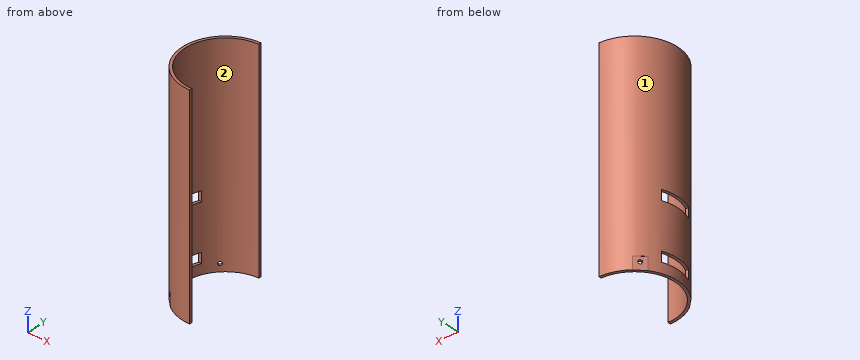
```python
from build123d import *

# Parameters (mm, degrees)
BOSS_EXTRUDE1_DEPTH      = 250
M4_CLEARANCE_HOLE1_D     = 4.5
M4_CLEARANCE_HOLE1_DEPTH = 15
M4_CLEARANCE_HOLE1_TIP   = 1.351936393
M4_CLEARANCE_HOLE2_D     = 4.5
M4_CLEARANCE_HOLE2_DEPTH = 15
M4_CLEARANCE_HOLE2_TIP   = 1.351936393
SKETCH9_W                = 12
SKETCH9_H                = 19.5
CUT_EXTRUDE1_DEPTH       = 10
CUT_EXTRUDE2_DEPTH       = 15
CIRPATTERN1_COUNT        = 2
CIRPATTERN1_ANGLE        = 270
CUT_EXTRUDE4_DEPTH       = 251.0000001


with BuildPart() as part:
    # Sketch1 → Boss-Extrude1 (new body)
    with BuildSketch(Plane.XY):
        with BuildLine():
            Line((0, 50.8), (0, 47.62))
            ThreePointArc((0, 47.62), (-47.62, 0), (0, -47.62))
            Line((0, -47.62), (0, -50.8))
            ThreePointArc((0, -50.8), (-50.8, 0), (0, 50.8))
        make_face()
    extrude(amount=BOSS_EXTRUDE1_DEPTH)

    # M4 Clearance Hole1
    with Locations(Plane(origin=(-35.921024484, 35.921024484, 0), x_dir=(0, 0, -1), z_dir=(-0.707106781, 0.707106781, 0))):
        with Locations((-9, 0)):
            Hole(M4_CLEARANCE_HOLE1_D / 2, depth=M4_CLEARANCE_HOLE1_DEPTH)
            with Locations((0, 0, -(M4_CLEARANCE_HOLE1_DEPTH + M4_CLEARANCE_HOLE1_TIP / 2))):  # 118° drill point
                Cone(0, M4_CLEARANCE_HOLE1_D / 2, M4_CLEARANCE_HOLE1_TIP, mode=Mode.SUBTRACT)

    # M4 Clearance Hole2
    with Locations(Plane(origin=(-35.921024484, -35.921024484, 0), x_dir=(0, 0, -1), z_dir=(-0.707106781, -0.707106781, 0))):
        with Locations((-9, 0)):
            Hole(M4_CLEARANCE_HOLE2_D / 2, depth=M4_CLEARANCE_HOLE2_DEPTH)
            with Locations((0, 0, -(M4_CLEARANCE_HOLE2_DEPTH + M4_CLEARANCE_HOLE2_TIP / 2))):  # 118° drill point
                Cone(0, M4_CLEARANCE_HOLE2_D / 2, M4_CLEARANCE_HOLE2_TIP, mode=Mode.SUBTRACT)

    # Sketch9 → Cut-Extrude1 (cut)
    with BuildSketch(Plane.ZY.offset(50.8)):
        with Locations((84, 9.75)):
            Rectangle(SKETCH9_W, SKETCH9_H)
        with Locations((84, -9.75)):
            Rectangle(SKETCH9_W, SKETCH9_H)
        Polygon((12, -19.5), (12, 0), (12, 19.5), (24, 19.5), (24, -19.5), align=None)
    extrude(amount=-CUT_EXTRUDE1_DEPTH, mode=Mode.SUBTRACT)

    # Sketch14 → Cut-Extrude2 (cut)
    with BuildSketch(Plane(origin=(0, 0, 0), x_dir=(-1, 0, 0), z_dir=(0, 0, -1))):
        with BuildLine():
            ThreePointArc((39.283322842, 32.206077218), (37.648654114, 34.102634894), (35.922518496, 35.916340685))
            Line((35.922518496, 35.916340685), (35.747788936, 35.741611124))
            Line((35.747788936, 35.741611124), (39.283322842, 32.206077218))
        make_face()
        with BuildLine():
            Line((35.747788936, 35.741611124), (35.922518496, 35.916340685))
            ThreePointArc((35.922518496, 35.916340685), (34.105872379, 37.645721305), (32.206077218, 39.283322842))
            Line((32.206077218, 39.283322842), (35.747788936, 35.741611124))
        make_face()
        with BuildLine():
            ThreePointArc((40.594896689, 30.540045233), (38.353880463, 33.310956958), (35.924113257, 35.917935446))
            Line((35.924113257, 35.917935446), (35.922518496, 35.916340685))
            ThreePointArc((35.922518496, 35.916340685), (37.648654114, 34.102634894), (39.283322842, 32.206077218))
            Line((39.283322842, 32.206077218), (35.747788936, 35.741611124))
            Line((35.747788936, 35.741611124), (35.570559867, 35.564382055))
            Line((35.570559867, 35.564382055), (40.594896689, 30.540045233))
        make_face()
        with BuildLine():
            Line((35.922518496, 35.916340685), (35.924113257, 35.917935446))
            ThreePointArc((35.924113257, 35.917935446), (33.314254946, 38.351015859), (30.540045233, 40.594896689))
            Line((30.540045233, 40.594896689), (35.570559867, 35.564382055))
            Line((35.570559867, 35.564382055), (35.747788936, 35.741611124))
            Line((35.747788936, 35.741611124), (32.206077218, 39.283322842))
            ThreePointArc((32.206077218, 39.283322842), (34.105872379, 37.645721305), (35.922518496, 35.916340685))
        make_face()
    cut_extrude2 = extrude(amount=-CUT_EXTRUDE2_DEPTH, mode=Mode.SUBTRACT)

    # CirPattern1: Cut-Extrude2 ×2 about axis
    cirpattern1_axis = Axis((0, 0, 250), (0, 0, -1))
    for i in range(1, CIRPATTERN1_COUNT):
        add(cut_extrude2.rotate(cirpattern1_axis, i * CIRPATTERN1_ANGLE / (CIRPATTERN1_COUNT - 1)), mode=Mode.SUBTRACT)

    # Sketch15 → Cut-Extrude4 (cut, through all)
    with BuildSketch(Plane(origin=(0, 0, 0), x_dir=(-1, 0, 0), z_dir=(0, 0, -1))):
        Polygon((0, 50.8), (0.15, 50.8), (0.15, -50.799778543), (0.15, -50.826071735), (0, -50.826071735), (0, -50.799778543), align=None)
    extrude(amount=-CUT_EXTRUDE4_DEPTH, mode=Mode.SUBTRACT)


solid = part.part
```
The model under review builds one solid part; all positions refer to its coordinate system, in mm. Face numbers are marked on the shaded views. Round coordinates to 2 decimals unless told otherwise and drop trailing zeros. Order: outer loops, then holes, each group sorted by start corner. A loop starts at its lowest first (then second) coordinate and runs counter-clockwise, first axis right, second up.
Item 1: Add section B-B, the plane x = -9. State the section outline as (y, z) points.
Working result:
outline: (-50, 0) - (-46.76, 0) - (-46.76, 250) - (-50, 250) - close; (46.76, 0) - (50, 0) - (50, 250) - (46.76, 250) - close
Item 2: Add section C-C, the plane z = 125.5. State the section outline as (x, y) points.
Working result:
outline: (-0.15, -50.8) - (-0.15, -47.62) arc R47.62 cw to (-0.15, 47.62) - (-0.15, 50.8) arc R50.8 ccw to start
Item 3: Add section A-A, the plane y = 0. State the section outline as (x, z) points.
Working result:
outline: (-50.8, 0) - (-47.62, 0) - (-47.62, 12) - (-50.8, 12) - close; (-50.8, 24) - (-47.62, 24) - (-47.62, 78) - (-50.8, 78) - close; (-50.8, 90) - (-47.62, 90) - (-47.62, 250) - (-50.8, 250) - close
Item 4: For pin 1 (10 mm diameter, centred on y = 26.5, z = 44, fed in from +X); pin 2 (1.5 mm diameter, centred on y = 9.5, z = 198.5, fed in from -X); pin 3 (11 mm diameter, centred on x = -34.5, y = -37.5, fed in from -Z); pin 4 (4 mm diameter, centred on x = -45, z = 16, fed in from -Y), all flat-tipped, find the tip position at first contact; note any pin that passes through.
Working result:
pin 1: stops at x = -35.71
pin 2: stops at x = -50.04
pin 3: stops at z = 0
pin 4: stops at y = -27.05
Item 5: Draft analysis for pull direction Y (two halves, no side actions). For the marked faces 1 and 2, state which applies: released by +Y, released by -Y, zero draft, split by the parting line, or undercut.
Working result:
face 1: split by the parting line
face 2: undercut
Item 6: To check wall thickness, follow probe 1 along Z at (x, y) = (-45.5, -15); probe 2 along Y at (x, z) = (-28, 168); probe 3 along Y at (x, z) = (-27.5, 86). State the ranges of each line that lie inside material, in increasing order.
Working result:
probe 1: z = 0 to 12, 24 to 78, 90 to 250
probe 2: y = -42.39 to -38.52, 38.52 to 42.39
probe 3: y = -42.71 to -38.88, 38.88 to 42.71
